from build123d import *

# Parameters (mm, degrees)
F0_W     = 66.9934824109
F0_H     = 90.5065238476
F1_DEPTH = 25
F2_W     = 16.0485785455
F2_H     = 76.6972787678
F3_DEPTH = 25.001
F5_DEPTH = 25.001
F6_W     = 21.2736960966
F6_H     = 12.6895736903
F7_DEPTH = 25.001
F8_W     = 8.3975102752
F8_H     = 13.8092450798
F9_DEPTH = 25.001


with BuildPart() as f1:
    # F0 (on Top) → F1 (new body)
    with BuildSketch(Plane.XY):
        Rectangle(F0_W, F0_H)
    extrude(amount=F1_DEPTH)

    # F2 (on face) → F3 (cut, through all)
    with BuildSketch(Plane.XY.offset(25)):
        with Locations((25.4724519327, 6.9046225399)):
            Rectangle(F2_W, F2_H)
    extrude(amount=-F3_DEPTH, mode=Mode.SUBTRACT)

    # F4 (on face) → F5 (cut, through all)
    with BuildSketch(Plane.XY.offset(25)):
        Polygon((-33.4967412055, 22.3143491894), (-15.9534495324, 45.2532619238), (-33.4967412055, 45.2532619238), align=None)
        Polygon((17.44816266, 45.2532619238), (2.3326422088, 45.2532619238), (17.44816266, 27.7117881924), align=None)
    extrude(amount=-F5_DEPTH, mode=Mode.SUBTRACT)

    # F6 (on face) → F7 (cut, through all)
    with BuildSketch(Plane.XY.offset(25)):
        with Locations((6.8113146117, -25.0992299989)):
            Rectangle(F6_W, F6_H)
    extrude(amount=-F7_DEPTH, mode=Mode.SUBTRACT)

    # F8 (on face) → F9 (cut, through all)
    with BuildSketch(Plane.XY.offset(25)):
        with Locations((29.2979860678, -38.3486393839)):
            Rectangle(F8_W, F8_H)
    extrude(amount=-F9_DEPTH, mode=Mode.SUBTRACT)


solid = f1.part
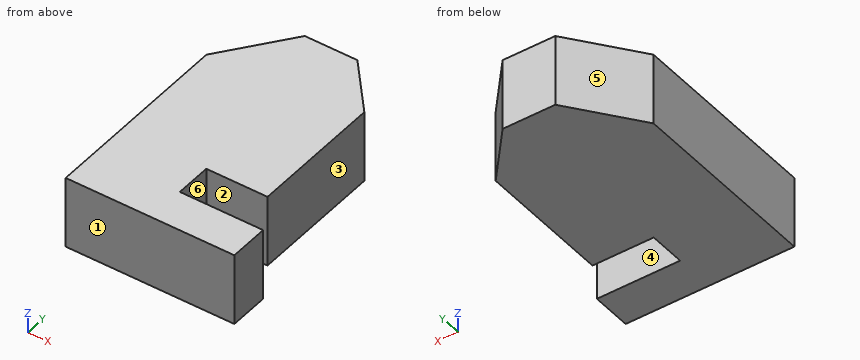
Build history of the part. All positions in model axes, mm. Face numbers are marked on the shaded views. A direction names the side the tool comes from. Coordinates: 2 decimals unless noted, no trailing zeros. Order: outer loops, then holes, each group sorted by start corner. A loop starts at its lowest first (then second) coordinate and runs counter-clockwise, first axis right, second up. Notation, with made-up numbers: (24, 14) - (73, 14) arc R25 ccw to (73, 33) - close; hole circle Ø6 at (44, 39.5). An arc over 180 degrees is marked (long way). Write each question's results on one line, items separated by ' | '. Start each with the question number.
Item 1: Band-saw the part on A-A on z = 8.5. Write the cut outline in (x, y).
Item 2: Flat gauge pins, fed straight in: pin 1 (1.5 mm diameter, centred on y = -5.5, z = 16.5, fed in from +X); pin 2 (1.5 mm diameter, centred on y = -26, z = 11, fed in from +X). Where does each tip first touch, or does it go through?
Item 3: Band-saw the part on C-C on y = -10. Write the cut outline in (x, z), and give its area (3 significant figures).
Item 4: Wall check: probe 1 along Y at (x, z) = (1, 23.75); probe 2 along Y at (x, z) = (23.5, 6); probe 3 along X at (y, z) = (-1, 10). Give the ranges that are in metal, low to high. Write a range as [from, to].
Item 5: Band-saw the part on D-D on y = -26.5. Write the cut outline in (x, z), and give its area (3 significant figures).
Item 6: Band-saw the part on B-B on x = 3.5. Write the cut outline in (y, z).
Item 7: Tool access for the marked faces 5 and 6: list every direction of +Z, -Z, +X, -X, +Y, -Y with a clear straight run to the whole face (end or side of a thin tool).
Item 8: Mould opens along Y. For the marked faces 1, 2, 3 and 4 say: released by +Y, released by -Y, zero draft, split by the parting line, or undercut.
Numbers:
1) outline: (-33.5, -45.25) - (25.1, -45.25) - (25.1, -31.44) - (-3.83, -31.44) - (-3.83, -18.75) - (17.45, -18.75) - (17.45, 27.71) - (2.33, 45.25) - (-15.95, 45.25) - (-33.5, 22.31) - close
2) pin 1: x = 17.45 | pin 2: x = -3.83
3) outline: (-33.5, 0) - (17.45, 0) - (17.45, 25) - (-33.5, 25) - close | area: 1,270 mm^2
4) probe 1: [-45.25, -31.44], [-18.75, 45.25] | probe 2: [-45.25, -31.44] | probe 3: [-33.5, 17.45]
5) outline: (-33.5, 0) - (-3.83, 0) - (-3.83, 25) - (-33.5, 25) - close | area: 742 mm^2
6) outline: (-45.25, 0) - (-31.44, 0) - (-31.44, 25) - (-45.25, 25) - close; (-18.75, 0) - (43.9, 0) - (43.9, 25) - (-18.75, 25) - close
7) face 5: +Z, -Z, -X, +Y | face 6: +Z, -Z, +X
8) face 1: released by -Y | face 2: undercut | face 3: zero draft | face 4: undercut
